Autodesk Inventor part; units mm, degrees
ref_plane "YZ Plane" through (0, 0, 0) normal (1, 0, 0) x (0, 1, 0)
ref_plane "XZ Plane" through (0, 0, 0) normal (0, 1, 0) x (-1, 0, 0)
ref_plane "XY Plane" through (0, 0, 0) normal (0, 0, 1) x (1, 0, 0)
sketch "Skizze1" plane through (0, 0, 0) normal (0, 0, 1) x (1, 0, 0)
  line L0 (2.5, -1.4434) -> (0, -2.8868)
  line L1 (0, -2.8868) -> (-2.5, -1.4434)
  line L2 (-2.5, -1.4434) -> (-2.5, 1.4434)
  line L3 (-2.5, 1.4434) -> (0, 2.8868)
  line L4 (0, 2.8868) -> (2.5, 1.4434)
  line L5 (2.5, 1.4434) -> (2.5, -1.4434)
  line L6 (0, 4.4456) -> (0, -4.4456)
  point P0 (0, 0)
  point P1 (0, 0)
  dimension "SW" = 5
extrude "Extrusion1" add sketch "Skizze1" along normal mid plane 10
sketch "Skizze2" plane through (0, 0, 5) normal (0, 0, 1) x (1, 0, 0)
  point P0 (0, 0)
  point P1 (0, 0)
hole "Bohrung1" at (0, 0, 5) direction (0, 0, -1) diameter 2.013 depth 7 tip angle 118
sketch "Skizze3" plane through (0, 0, -5) normal (0, 0, -1) x (-1, 0, 0)
  circle A0 centre (0, 0) radius 1.25
  dimension "GA_" = 2.5
extrude "Extrusion2" add sketch "Skizze3" along normal blind 6
thread "Gewinde1"
chamfer "Fase1" distance 0.25 angle 45 1 edges at (1.25, 0, -11)
sketch "Skizze4" plane through (0, 0, 5) normal (0, 0, 1) x (1, 0, 0)
  line L0 (2.5, -1.4434) -> (2.5, 1.4434)
  circle A0 centre (0, 0) radius 2.5
sketch "Skizze5" plane through (0, 0, 0) normal (1, 0, 0) x (0, 1, 0)
  line L0 (-1.0065, 5) -> (1.0065, 5)
  line L1 (-2.8868, 5) -> (-1.4434, 5)
  line L2 (-1.4434, 5) -> (1.4434, 5)
  line L3 (1.4434, 5) -> (2.8868, 5)
  line L4 (2.8868, 5) -> (1.4434, 5)
  line L5 (1.4434, 5) -> (-1.4434, 5)
  line L6 (-1.4434, 5) -> (-2.8868, 5)
  line L7 (2.5, 5) -> (-2.5, 5)
  line L8 (2.8868, 5) -> (2.5, 5)
  line L9 (2.5, 5) -> (2.8868, 4.6132)
  line L10 (2.8868, 4.6132) -> (2.8868, 5)
  line L11 (0, 7) -> (0, -7)
  line L12 (1.25, -5) -> (-1.25, -5)
  line L13 (-1.4434, -5) -> (-2.8868, -5)
  line L14 (-2.8868, -5) -> (-1.4434, -5)
  line L15 (-1.4434, -5) -> (1.4434, -5)
  line L16 (1.4434, -5) -> (2.8868, -5)
  line L17 (2.8868, -5) -> (1.4434, -5)
  line L18 (1.4434, -5) -> (-1.4434, -5)
  line L19 (0, 5) -> (0, -5)
  point P0 (0, 0)
  dimension "d20" = 45
revolve "Umdrehung1" cut sketch "Skizze5" angle 360 about axis through (0, 0, 5) along (0, 0, -1)
mirror "Spiegeln1" about plane through (0, 0, 0) normal (0, 0, 1) of "Umdrehung1"
properties part number "M2.5" material "Stahl"
Source: CAD feature listing. Evaluate the final solid. Frame: model axes, mm. A direction names the side the tool comes from. Round coordinates to 2 decimals unless told otherwise and drop trailing zeros. Loops run counter-clockwise (first coordinate to the right, second up) from the corner with the lowest first, then second, coordinate; pieces in that order, holes last.
1. Contact query for flat-ended pins moving along their axis: pin 1 (1.5 mm diameter, centred on y = 2, z = -5.5, fed in from -X); pin 2 (1 mm diameter, centred on x = -0.5, y = -2.5, fed in from -Z); pin 3 (1 mm diameter, centred on y = -2, z = -5, fed in from -X). Output: stop coordinate, or through.
2. Section query A-A on z = 2.75. Output: boundary loops of the cut face in (x, y).
3. Ray query, L1, parallel to X at y = 0, z = 2.5; L2, parallel to Z at x = -1.75, y = 1.15; L3, parallel to Y at x = 0.55, z = -1. Return the intervals inside material, ascending.
4. Access query for faces 1 (the flat face through (1, 1, -5)), 2 (the flat face through (1.268, -2.155, -0.07)). Directions: +Z, -Z, +X, -X, +Y, -Y. A direction counts if a zero-diameter tool reaches every point of the face in a straight line with its end or side. Return the directions, or none.
5. Mould query, pull axis X, two halves, no side actions, for faces 3 (the cylindrical face through (0.983, 0.218, 1.451)), 4 (the flat face through (1, -1, 5)), 5 (the conical face through (-0.06, -2.61, -4.89)). Classes: released by +X, released by -X, zero draft, split by the parting line, or undercut.
Answers below:
1. pin 1: stops at x = -2.09
1. pin 2: stops at z = -5
1. pin 3: stops at x = -2.27
2. outline: (-2.5, -1.44) - (0, -2.89) - (2.5, -1.44) - (2.5, 1.44) - (0, 2.89) - (-2.5, 1.44) - close; hole circle Ø2.01 at (0, 0)
3. L1: x = -2.5 to -1.01, 1.01 to 2.5
3. L2: z = -5 to 5
3. L3: y = -2.57 to -0.84, 0.84 to 2.57
4. face 1: -Z
4. face 2: +Z, -Z, +X, -Y
5. face 3: undercut
5. face 4: zero draft
5. face 5: split by the parting line
